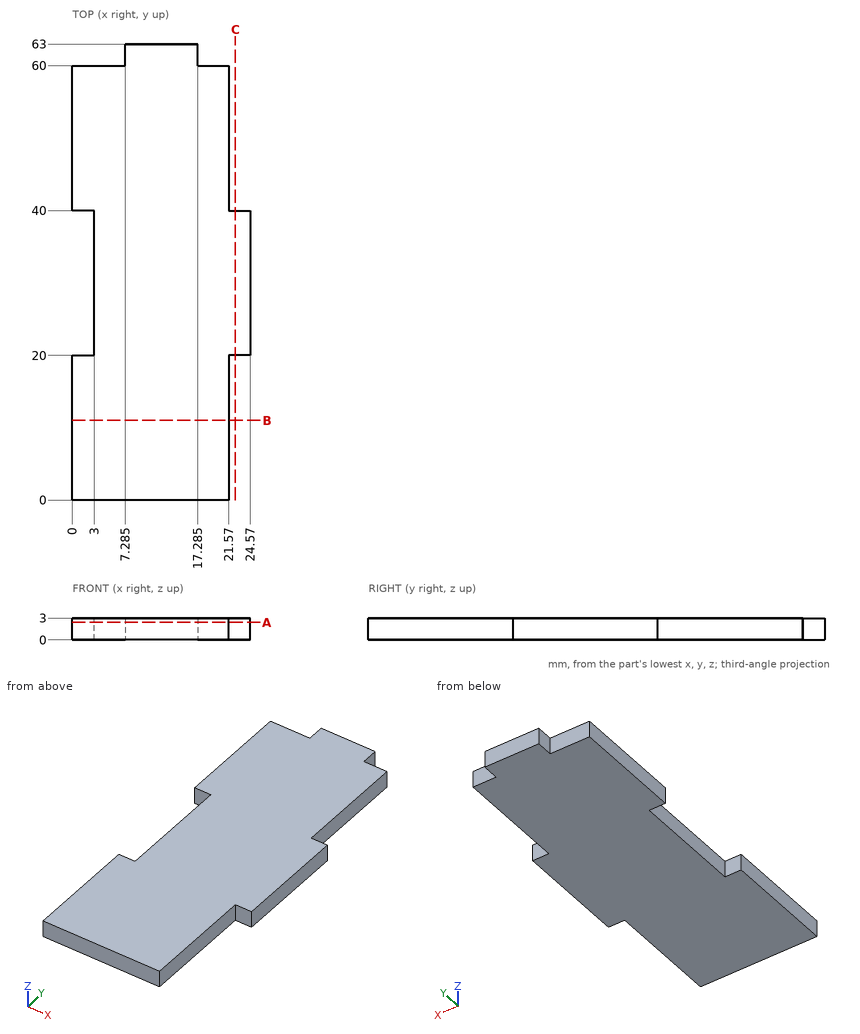
Job drawing, mm, ordinate dimensions from the low corner. One solid piece. Round coordinates to 2 decimals unless told otherwise and drop trailing zeros. Order: outer loops, then holes, each group sorted by start corner. A loop starts at its lowest first (then second) coordinate and runs counter-clockwise, first axis right, second up. Notation, with made-up numbers: (37.25, 84) -> (46.25, 84) arc R20 ccw to (46.25, 120) -> close; hole circle Ø7 at (85.5, 50.25). An arc over 180 degrees is marked (long way). Write item = value, one per line.
(1) Cut at B-B (y = 11). Write the cut outline in (x, z), plus the area to 3 significant figures.
Answers follow:
outline = (0, 0) -> (21.57, 0) -> (21.57, 3) -> (0, 3) -> close
area = 64.7 mm²
(2) Drill centre lines: L1, parallel to Y at x = 4.5, z = 2.8; L2, parallel to X at y = 60.5, z = 0.25 (3 decimals); L3, parallel to X at y = 59.5, z = 0.8. Where is each one in solid material? Low to high.
Answers follow:
L1 = 0 to 60
L2 = 7.285 to 17.285
L3 = 0 to 21.57
(3) Cut at C-C (x = 22.5). Write the cut outline in (y, z), plus the area to 3 significant figures.
Answers follow:
outline = (20, 0) -> (40, 0) -> (40, 3) -> (20, 3) -> close
area = 60.0 mm²
(4) Cut at A-A (z = 2.4). Write the cut outline in (x, y) (3 decimals).
Answers follow:
outline = (0, 0) -> (21.57, 0) -> (21.57, 20) -> (24.57, 20) -> (24.57, 40) -> (21.57, 40) -> (21.57, 60) -> (17.285, 60) -> (17.285, 63) -> (7.285, 63) -> (7.285, 60) -> (0, 60) -> (0, 40) -> (3, 40) -> (3, 20) -> (0, 20) -> close
(5) Flat gauge pins, fed straight in: P1, Ø0.9, axis at x = 20.5, z = 1.5, coming from the +Y side; P2, Ø0.9, axis at y = 9.5, z = 1.5, coming from the +X side; P3, Ø1.5, axis at x = 23, z = 1.5, coming from the +Y side. Where does each tip first touch, or does it go through?
Answers follow:
P1 = 60
P2 = 21.57
P3 = 40
